The listing builds one solid part. Answer for the finished solid, in the listing's coordinates (mm). A direction names the side the tool comes from. Round coordinates to 2 decimals unless told otherwise and drop trailing zeros. Write each loop counter-clockwise with the first axis right and the second up, starting at its lowest first coordinate (ties: lowest second). Pieces come first, ordered by that corner, then holes. Notation, with made-up numbers: (-11, 86.25) - (22, 86.25) arc R23 cw to (22, 120.25) - close; hole circle Ø2 at (80.5, 49.25). An arc over 180 degrees is marked (long way). Answer in a Markdown table with one row per item.
from build123d import *

# Parameters (mm, degrees)
F0_R      = 77.5
F0_R_2    = 75
F1_DEPTH  = 70
F2_R      = 1
F3_DEPTH  = 3
F4_R      = 30
F4_R_2    = 27
F5_DEPTH  = 10
F7_DEPTH  = 10
F10_DEPTH = 17
F12_R     = 10


with BuildPart() as f1:
    # F0 (on Top) → F1 (new body)
    with BuildSketch(Plane.XY):
        Circle(F0_R)
        Circle(F0_R_2, mode=Mode.SUBTRACT)
    extrude(amount=F1_DEPTH)


with BuildPart() as f3:
    # F2 (on Top) → F3 (new body)
    with BuildSketch(Plane.XY):
        with BuildLine():
            Line((8.3085046789, -8.3085046789), (28.8265285805, -8.3085046789))
            ThreePointArc((28.8265285805, -8.3085046789), (30, 0), (28.8265285805, 8.3085046789))
            Line((28.8265285805, 8.3085046789), (8.3085046789, 8.3085046789))
            Line((8.3085046789, 8.3085046789), (8.3085046789, 28.8265285805))
            ThreePointArc((8.3085046789, 28.8265285805), (0, 30), (-8.3085046789, 28.8265285805))
            Line((-8.3085046789, 28.8265285805), (-8.3085046789, 8.3085046789))
            Line((-8.3085046789, 8.3085046789), (-28.8265285805, 8.3085046789))
            ThreePointArc((-28.8265285805, 8.3085046789), (-30, 0), (-28.8265285805, -8.3085046789))
            Line((-28.8265285805, -8.3085046789), (-8.3085046789, -8.3085046789))
            Line((-8.3085046789, -8.3085046789), (-8.3085046789, -28.8265285805))
            ThreePointArc((-8.3085046789, -28.8265285805), (0, -30), (8.3085046789, -28.8265285805))
            Line((8.3085046789, -28.8265285805), (8.3085046789, -8.3085046789))
        make_face()
        with Locations((0, -16.6170093579)):
            Circle(F2_R, mode=Mode.SUBTRACT)
        with Locations((-16.6170093579, 0)):
            Circle(F2_R, mode=Mode.SUBTRACT)
        with BuildLine():
            ThreePointArc((15.6170093579, 0), (16.6170093579, 1), (17.6170093579, 0))
            ThreePointArc((17.6170093579, 0), (16.6170093579, -1), (15.6170093579, 0))
        make_face(mode=Mode.SUBTRACT)
        with Locations((0, 16.6170093579)):
            Circle(F2_R, mode=Mode.SUBTRACT)
    extrude(amount=F3_DEPTH)

    # F4 (on Top) → F5 (join)
    with BuildSketch(Plane.XY):
        Circle(F4_R)
        Circle(F4_R_2, mode=Mode.SUBTRACT)
    extrude(amount=F5_DEPTH)


with BuildPart() as f7:
    # F6 (on Top) → F7 (new body)
    with BuildSketch(Plane.XY):
        with BuildLine():
            Line((-19.3094096744, -22.9596754774), (-22.9596754774, -19.3094096744))
            ThreePointArc((-22.9596754774, -19.3094096744), (-21.2132034356, -21.2132034356), (-19.3094096744, -22.9596754774))
        make_face()
        with BuildLine():
            ThreePointArc((-19.3094096744, -22.9596754774), (-21.2132034356, -21.2132034356), (-22.9596754774, -19.3094096744))
            Line((-22.9596754774, -19.3094096744), (-54.8267261784, -51.1764603754))
            Line((-54.8267261784, -51.1764603754), (-51.1764603754, -54.8267261784))
            Line((-51.1764603754, -54.8267261784), (-19.3094096744, -22.9596754774))
        make_face()
        with BuildLine():
            Line((-51.1764603754, -54.8267261784), (-54.8267261784, -51.1764603754))
            ThreePointArc((-54.8267261784, -51.1764603754), (-53.033008589, -53.033008589), (-51.1764603754, -54.8267261784))
        make_face()
    extrude(amount=F7_DEPTH)


with BuildPart() as f7b:
    # F6 (on Top) → F7, piece 2 (new body)
    with BuildSketch(Plane.XY):
        with BuildLine():
            ThreePointArc((51.1764603754, -54.8267261784), (53.033008589, -53.033008589), (54.8267261784, -51.1764603754))
            Line((54.8267261784, -51.1764603754), (22.9596754774, -19.3094096744))
            ThreePointArc((22.9596754774, -19.3094096744), (21.2132034356, -21.2132034356), (19.3094096744, -22.9596754774))
            Line((19.3094096744, -22.9596754774), (51.1764603754, -54.8267261784))
        make_face()
    extrude(amount=F7_DEPTH)


with BuildPart() as f7c:
    # F6 (on Top) → F7, piece 3 (new body)
    with BuildSketch(Plane.XY):
        with BuildLine():
            ThreePointArc((-51.1764603754, 54.8267261784), (-53.033008589, 53.033008589), (-54.8267261784, 51.1764603754))
            Line((-54.8267261784, 51.1764603754), (-22.9596754774, 19.3094096744))
            ThreePointArc((-22.9596754774, 19.3094096744), (-21.2132034356, 21.2132034356), (-19.3094096744, 22.9596754774))
            Line((-19.3094096744, 22.9596754774), (-51.1764603754, 54.8267261784))
        make_face()
    extrude(amount=F7_DEPTH)


with BuildPart() as f7d:
    # F6 (on Top) → F7, piece 4 (new body)
    with BuildSketch(Plane.XY):
        Polygon((14.0217830061, 26.418115506), (26.418115506, 14.0217830061), (59.726265439, 47.3299329391), (47.3299329391, 59.726265439), align=None)
    extrude(amount=F7_DEPTH)


with BuildPart() as f10_tool:
    # F9 (on offset) → F10 (new body)
    with BuildSketch(Plane.XY.offset(20)):
        Polygon((13.2823127623, 21.2434951856), (21.2434951856, 13.2823127623), (60.5607913141, 52.5996088908), (52.5996088908, 60.5607913141), align=None)
    extrude(amount=-F10_DEPTH)


with BuildPart() as f1_1:
    add(f1.part)

    # F10: cut by f10_tool
    add(f10_tool.part, mode=Mode.SUBTRACT)


with BuildPart() as f3_1:
    add(f3.part)

    # F10: cut by f10_tool
    add(f10_tool.part, mode=Mode.SUBTRACT)


with BuildPart() as f7d_1:
    add(f7d.part)

    # F10: cut by f10_tool
    add(f10_tool.part, mode=Mode.SUBTRACT)


with BuildPart() as f3_2:
    add(f3_1.part)

    # F11: union F7, F7b, F7c, F7d, F1
    add(f7.part)
    add(f7b.part)
    add(f7c.part)
    add(f7d_1.part)
    add(f1_1.part)

    # F12
    f12_edges = [f3_2.edges().sort_by_distance(p)[0] for p in [
        (-51.17646, 54.826726, 5),
        (-54.826726, 51.17646, 5),
        (58.867728, 46.471396, 5),
        (46.471396, 58.867728, 5),
        (51.17646, -54.826726, 5),
        (54.826726, -51.17646, 5),
        (-51.17646, -54.826726, 5),
        (-54.826726, -51.17646, 5),
        (-22.959675, -19.30941, 5),
        (-19.30941, -22.959675, 5),
        (22.959675, -19.30941, 5),
        (14.089336, 26.485668, 5),
        (26.485668, 14.089336, 5),
        (-19.30941, 22.959675, 5),
        (-22.959675, 19.30941, 5),
    ]]
    fillet(f12_edges, radius=F12_R)


solid = f3_2.part
(1) Find the intervals of material crossed by line 1 (Y direction, x = 0, z = 0.7); line 2 (Y direction, x = -34.5, z = 7.5); line 3 (X direction, y = 49, z = 43.5), in increasing order.
Checked values:
| item | result |
|---|---|
| line 1 | y = -77.5 to -75, -30 to -17.62, -15.62 to 15.62, 17.62 to 30, 75 to 77.5 |
| line 2 | y = -69.4 to -66.59, -38.15 to -30.85, 30.85 to 38.15, 66.59 to 69.4 |
| line 3 | x = -60.04 to -56.78, 56.78 to 60.04 |
(2) For a pull along X with two mould halves and no side action, classify faces 1 (the flat face through (-41, 64, 70)), 2 (the cylindrical face through (54.84, -46.16, 5.07)), 3 (the cylindrical face through (-16.8, -75.657, 34.51)) as pulls with the +X half, pulls with the -X half, needs draft (parallel to the pull), parting line crosses it, or undercut.
Checked values:
| item | result |
|---|---|
| face 1 | needs draft |
| face 2 | undercut |
| face 3 | parting line crosses it |
(3) Section A-A (y = 4) is taken. Give the vertices of the cut face in (x, z).
Checked values:
| item | result |
|---|---|
| outline | (-77.4, 0) - (-74.89, 0) - (-74.89, 70) - (-77.4, 70) - close; (-29.73, 0) - (29.73, 0) - (29.73, 10) - (26.7, 10) - (26.7, 3) - (-26.7, 3) - (-26.7, 10) - (-29.73, 10) - close; (74.89, 0) - (77.4, 0) - (77.4, 70) - (74.89, 70) - close |
(4) Section B-B (y = -66) is taken. Give the vertices of the cut face in (x, z), and give its area (3 significant figures).
Checked values:
| item | result |
|---|---|
| outline | (-40.62, 0) - (-35.62, 0) - (-35.62, 70) - (-40.62, 70) - close; (35.62, 0) - (40.62, 0) - (40.62, 70) - (35.62, 70) - close |
| area | 700 mm2 |
(5) Flat-ended cylindrical pins translate along their axes: pin 1 (3 mm diameter, centred on x = 53.5, y = -57, fed in from +Z); pin 2 (0.9 mm diameter, centred on x = 20, z = 1, fed in from +Y); pin 3 (3.5 mm diameter, centred on y = 14.5, z = 1, fed in from +X); pin 4 (10 mm diameter, centred on x = 12.5, z = 59, fed in from -Y). Find the tip coordinate at first contact, or state that the pin passes through.
Checked values:
| item | result |
|---|---|
| pin 1 | stops at z = 70 |
| pin 2 | stops at y = 74.99 |
| pin 3 | stops at x = 76.44 |
| pin 4 | stops at y = -77.14 |
(6) Section C-C (z = 60) is taken. Give the vertices of the cut face in (x, y), and give its area (3 significant figures).
Checked values:
| item | result |
|---|---|
| outline | circle Ø155 at (0, 0); hole circle Ø150 at (0, 0) |
| area | 1,200 mm2 |
(7) For faces 4 (the cylindrical face through (-2.363, 29.907, 4.93)), 5 (the flat face through (32.94, 40.9, 7.84)), 6 (the cylindrical face through (69.28, -28.73, 34.51)), determine the directions among +Z, -Z, +X, -X, +Y, -Y from which every point of the face is accessible in a straight line to the end or side of a thin tool.
Checked values:
| item | result |
|---|---|
| face 4 | +Z, -Z |
| face 5 | none |
| face 6 | +Z |
